```python
from build123d import *

# Parameters (mm, degrees)
SKETCH1_W                                     = 1219.2
SKETCH1_H                                     = 1778
SKETCH1_R                                     = 254
SKETCH1_W_2                                   = 361.95
SKETCH1_H_2                                   = 361.95
BOSS_EXTRUDE1_DEPTH                           = 6.35
SKETCH3_R                                     = 209.55
CUT_EXTRUDE2_DEPTH                            = 7.35
SKETCH2_W                                     = 203.2
SKETCH2_H                                     = 165.1
CUT_EXTRUDE1_DEPTH                            = 7.35
SKETCH4_R                                     = 3.3655
CUT_EXTRUDE3_DEPTH                            = 7.35
LPATTERN1_COUNT                               = 5
LPATTERN1_PITCH                               = 425.45
SKETCH5_R                                     = 3.429
CUT_EXTRUDE4_DEPTH                            = 7.35
LPATTERN2_COUNT                               = 3
LPATTERN2_PITCH                               = 301.625
SKETCH6_R                                     = 3.96875
CUT_EXTRUDE5_DEPTH                            = 7.35
SKETCH7_R                                     = 3.3782
CUT_EXTRUDE6_DEPTH                            = 7.35
CSK_FOR_1_4_FLAT_HEAD_MACHINE_SCREW1_AT_COUNT = 2
CSK_FOR_1_4_FLAT_HEAD_MACHINE_SCREW1_AT_PITCH = 63.5
LPATTERN3_COUNT                               = 2
LPATTERN3_PITCH                               = 901.7
SKETCH12_R                                    = 4.7625
CUT_EXTRUDE7_DEPTH                            = 7.35
SKETCH14_R                                    = 4.7625
CUT_EXTRUDE8_DEPTH                            = 7.35
SKETCH15_R                                    = 4.7625
CUT_EXTRUDE9_DEPTH                            = 7.35
SKETCH16_R                                    = 4.7625
CUT_EXTRUDE10_DEPTH                           = 7.35
FILLET1_R                                     = 12.7
FILLET2_R                                     = 6.35
SKETCH17_R                                    = 3.937
CUT_EXTRUDE11_DEPTH                           = 7.35
CSK_FOR_1_4_FLAT_HEAD_MACHINE_SCREW2_AT_COUNT = 2
CSK_FOR_1_4_FLAT_HEAD_MACHINE_SCREW2_AT_PITCH = 95.25
CSK_FOR_1_4_FLAT_HEAD_MACHINE_SCREW2_2_COUNT  = 2
CSK_FOR_1_4_FLAT_HEAD_MACHINE_SCREW2_2_PITCH  = 381
CSK_FOR_1_4_FLAT_HEAD_MACHINE_SCREW2_3_COUNT  = 2
CSK_FOR_1_4_FLAT_HEAD_MACHINE_SCREW2_3_PITCH  = 392.72581084
F_5_16_0_3125_DIAMETER_HOLE1_D                = 7.9375


with BuildPart() as part:
    # Sketch1 → Boss-Extrude1 (new body)
    with BuildSketch(Plane.XY):
        with Locations((609.6, 889)):
            Rectangle(SKETCH1_W, SKETCH1_H)
        with Locations((330.2, 1473.2)):
            Circle(SKETCH1_R, mode=Mode.SUBTRACT)
        with Locations((609.6, 917.575)):
            Rectangle(SKETCH1_W_2, SKETCH1_H_2, mode=Mode.SUBTRACT)
    extrude(amount=BOSS_EXTRUDE1_DEPTH)

    # Sketch3 → Cut-Extrude2 (cut, through all)
    with BuildSketch(Plane.XY.offset(6.35)):
        with Locations((609.6, 279.4)):
            Circle(SKETCH3_R)
    extrude(amount=-CUT_EXTRUDE2_DEPTH, mode=Mode.SUBTRACT)

    # Sketch2 → Cut-Extrude1 (cut, through all)
    with BuildSketch(Plane.XY.offset(6.35)):
        with Locations((609.6, 44.45)):
            Rectangle(SKETCH2_W, SKETCH2_H)
        with Locations((609.6, 514.35)):
            Rectangle(SKETCH2_W, SKETCH2_H)
    extrude(amount=-CUT_EXTRUDE1_DEPTH, mode=Mode.SUBTRACT)

    # Sketch4 → Cut-Extrude3 (cut, through all)
    with BuildSketch(Plane.XY.offset(6.35)):
        with Locations((50.8, 12.7)):
            Circle(SKETCH4_R)
    cut_extrude3 = extrude(amount=-CUT_EXTRUDE3_DEPTH, mode=Mode.SUBTRACT)

    # LPattern1: Cut-Extrude3 ×5
    with Locations(*[(0, i * LPATTERN1_PITCH, 0) for i in range(1, LPATTERN1_COUNT)]):
        add(cut_extrude3, mode=Mode.SUBTRACT)

    # Sketch5 → Cut-Extrude4 (cut, through all)
    with BuildSketch(Plane.XY.offset(6.35)):
        with Locations((609.6, 1714.5)):
            Circle(SKETCH5_R)
    cut_extrude4 = extrude(amount=-CUT_EXTRUDE4_DEPTH, mode=Mode.SUBTRACT)

    # LPattern2: Cut-Extrude4 ×3
    with Locations(*[(0, -i * LPATTERN2_PITCH, 0) for i in range(1, LPATTERN2_COUNT)]):
        add(cut_extrude4, mode=Mode.SUBTRACT)

    # Sketch6 → Cut-Extrude5 (cut, through all)
    with BuildSketch(Plane.XY.offset(6.35)):
        with Locations((127, 12.7)):
            Circle(SKETCH6_R)
        with Locations((381, 12.7)):
            Circle(SKETCH6_R)
    extrude(amount=-CUT_EXTRUDE5_DEPTH, mode=Mode.SUBTRACT)

    # Sketch7 → Cut-Extrude6 (cut, through all)
    with BuildSketch(Plane.XY.offset(6.35)):
        with Locations((777.605208253, 88.9)):
            Circle(SKETCH7_R)
        with Locations((898.525, 342.9)):
            Circle(SKETCH7_R)
        with Locations((898.525, 215.9)):
            Circle(SKETCH7_R)
    extrude(amount=-CUT_EXTRUDE6_DEPTH, mode=Mode.SUBTRACT)

    # Sketch11 → CSK for 1/4 Flat Head Machine Screw1 (revolve, cut)
    with BuildSketch(Plane(origin=(127, 85.725, 6.35), x_dir=(0, -1, 0), z_dir=(1, 0, 0))):
        Polygon((0, 0), (0, 6.35), (3.57124, 6.35), (3.57124, 3.298865467), (6.4389, 0), align=None)
    csk_for_1_4_flat_head_machine_screw1 = revolve(axis=Axis((127, 85.725, 12.7), (0, 0, -1)), mode=Mode.SUBTRACT)

    # CSK for 1/4 Flat Head Machine Screw1 at: CSK for 1/4 Flat Head Machine Screw1 ×2
    with Locations(*[(i * CSK_FOR_1_4_FLAT_HEAD_MACHINE_SCREW1_AT_PITCH, 0, 0) for i in range(1, CSK_FOR_1_4_FLAT_HEAD_MACHINE_SCREW1_AT_COUNT)]):
        add(csk_for_1_4_flat_head_machine_screw1, mode=Mode.SUBTRACT)

    # LPattern3: CSK for 1/4 Flat Head Machine Screw1 ×2
    with Locations(*[(i * LPATTERN3_PITCH, 0, 0) for i in range(1, LPATTERN3_COUNT)]):
        add(csk_for_1_4_flat_head_machine_screw1, mode=Mode.SUBTRACT)

    # LPattern3 copy 1 sketch → LPattern3 copy 1 (revolve, cut)
    with BuildSketch(Plane(origin=(1092.2, 85.725, 6.35), x_dir=(0, -1, 0), z_dir=(1, 0, 0))):
        Polygon((0, 0), (0, 6.35), (3.57124, 6.35), (3.57124, 3.298865467), (6.4389, 0), align=None)
    revolve(axis=Axis((1092.2, 85.725, 12.7), (0, 0, -1)), mode=Mode.SUBTRACT)

    # Sketch12 → Cut-Extrude7 (cut, through all)
    with BuildSketch(Plane.XY.offset(6.35)):
        with Locations((203.2, 1727.2)):
            Circle(SKETCH12_R)
        with Locations((1016, 1727.2)):
            Circle(SKETCH12_R)
    extrude(amount=-CUT_EXTRUDE7_DEPTH, mode=Mode.SUBTRACT)

    # Sketch14 → Cut-Extrude8 (cut, through all)
    with BuildSketch(Plane.XY.offset(6.35)):
        with Locations((31.75, 1651)):
            Circle(SKETCH14_R)
        with Locations((31.75, 914.4)):
            Circle(SKETCH14_R)
        with Locations((31.75, 304.8)):
            Circle(SKETCH14_R)
    cut_extrude8 = extrude(amount=-CUT_EXTRUDE8_DEPTH, mode=Mode.SUBTRACT)

    # Mirror1: Cut-Extrude8 across plane
    add(cut_extrude8.mirror(Plane.ZY.offset(-609.6)), mode=Mode.SUBTRACT)

    # Sketch15 → Cut-Extrude9 (cut, through all)
    with BuildSketch(Plane.XY.offset(6.35)):
        with Locations((403.225, 736.6)):
            Circle(SKETCH15_R)
        with Locations((403.225, 682.625)):
            Circle(SKETCH15_R)
    cut_extrude9 = extrude(amount=-CUT_EXTRUDE9_DEPTH, mode=Mode.SUBTRACT)

    # Mirror2: Cut-Extrude9 across plane
    add(cut_extrude9.mirror(Plane.ZY.offset(-609.6)), mode=Mode.SUBTRACT)

    # Sketch16 → Cut-Extrude10 (cut, through all)
    with BuildSketch(Plane.XY.offset(6.35)):
        with Locations((419.1, 1054.1)):
            Circle(SKETCH16_R)
        with Locations((419.1, 787.4)):
            Circle(SKETCH16_R)
        with Locations((800.1, 1054.1)):
            Circle(SKETCH16_R)
        with Locations((800.1, 787.4)):
            Circle(SKETCH16_R)
    extrude(amount=-CUT_EXTRUDE10_DEPTH, mode=Mode.SUBTRACT)

    # Fillet1
    fillet1_edges = [part.edges().sort_by_distance(p)[0] for p in [
        (508, 0, 3.175),
        (711.2, 0, 3.175),
    ]]
    fillet(fillet1_edges, radius=FILLET1_R)

    # Fillet2
    fillet2_edges = [part.edges().sort_by_distance(p)[0] for p in [
        (428.625, 1098.55, 3.175),
        (428.625, 736.6, 3.175),
        (790.575, 736.6, 3.175),
        (790.575, 1098.55, 3.175),
        (711.2, 596.9, 3.175),
        (508, 596.9, 3.175),
        (0, 0, 3.175),
        (1219.2, 0, 3.175),
    ]]
    fillet(fillet2_edges, radius=FILLET2_R)

    # Sketch17 → Cut-Extrude11 (cut, through all)
    with BuildSketch(Plane.XY.offset(6.35)):
        with Locations((416.56762, 76.2)):
            Circle(SKETCH17_R)
        with Locations((416.56762, 19.05)):
            Circle(SKETCH17_R)
        with Locations((797.56762, 19.05)):
            Circle(SKETCH17_R)
        with Locations((797.56762, 76.2)):
            Circle(SKETCH17_R)
    extrude(amount=-CUT_EXTRUDE11_DEPTH, mode=Mode.SUBTRACT)

    # Sketch21 → CSK for 1/4 Flat Head Machine Screw2 (revolve, cut)
    with BuildSketch(Plane(origin=(418.15512, 576.972045059, 6.35), x_dir=(0, -1, 0), z_dir=(1, 0, 0))):
        Polygon((0, 0), (0, 6.35), (3.57124, 6.35), (3.57124, 3.298865467), (6.4389, 0), align=None)
    csk_for_1_4_flat_head_machine_screw2 = revolve(axis=Axis((418.15512, 576.972045059, 12.7), (0, 0, -1)), mode=Mode.SUBTRACT)

    # CSK for 1/4 Flat Head Machine Screw2 at: CSK for 1/4 Flat Head Machine Screw2 ×2
    with Locations(*[(0, -i * CSK_FOR_1_4_FLAT_HEAD_MACHINE_SCREW2_AT_PITCH, 0) for i in range(1, CSK_FOR_1_4_FLAT_HEAD_MACHINE_SCREW2_AT_COUNT)]):
        add(csk_for_1_4_flat_head_machine_screw2, mode=Mode.SUBTRACT)

    # CSK for 1_4 Flat Head Machine Screw2 2: CSK for 1/4 Flat Head Machine Screw2 ×2
    with Locations(*[(i * CSK_FOR_1_4_FLAT_HEAD_MACHINE_SCREW2_2_PITCH, 0, 0) for i in range(1, CSK_FOR_1_4_FLAT_HEAD_MACHINE_SCREW2_2_COUNT)]):
        add(csk_for_1_4_flat_head_machine_screw2, mode=Mode.SUBTRACT)

    # CSK for 1_4 Flat Head Machine Screw2 3: CSK for 1/4 Flat Head Machine Screw2 ×2
    with Locations(*[Vector(0.9701425, -0.242535625, 0) * (i * CSK_FOR_1_4_FLAT_HEAD_MACHINE_SCREW2_3_PITCH) for i in range(1, CSK_FOR_1_4_FLAT_HEAD_MACHINE_SCREW2_3_COUNT)]):
        add(csk_for_1_4_flat_head_machine_screw2, mode=Mode.SUBTRACT)

    # 5/16 (0.3125) Diameter Hole1 (through all)
    with Locations(Plane.XY.offset(6.35)):
        with Locations((334.9625, 68.2625), (334.9625, 14.2875), (884.2375, 14.2875), (884.2375, 68.2625)):
            Hole(F_5_16_0_3125_DIAMETER_HOLE1_D / 2)


solid = part.part
```
For this review, take the finished solid that the model builds, in its own axes (mm). A direction names the side the tool comes from. Round coordinates to 2 decimals unless told otherwise and drop trailing zeros. Write each question's results on one line, items separated by ' | '.
Item 1: Draft analysis for pull direction Y (two halves, no side actions). For faces 1 (the face through (400.073, 282.523, 3.219)), 2 (the face through (601, 704, 6.35)), state which applies: pulls with the +Y half, pulls with the -Y half, needs draft (parallel to the pull), parting line crosses it, or undercut.
Calculated:
face 1: undercut | face 2: needs draft
Item 2: For pin 1 (1.9 mm diameter, centred on x = 584.5, z = 3.5, fed in from -Y); pin 2 (11.5 mm diameter, centred on x = 418.16, y = 576.97, fed in from +Z), all flat-tipped, find the tip position at first contact; note any pin that passes through.
Calculated:
pin 1: stops at y = 596.9 | pin 2: stops at z = 5.56
Item 3: For faces 3 (the face through (819.127, 276.277, 3.219)), 4 (the face through (601, 704, 0)), list the 3-axis set-ups (+Z, -Z, +X, -X, +Y, -Y) from which the entire face can be reached by the end or side of a thin tool; tool diameter is ignored.
Calculated:
face 3: +Z, -Z | face 4: -Z, +X, -X, +Y, -Y
Item 4: Take a section at A-A on z = 5.25. Count the separate pieces of the cut face and the enclosed holes in it, then the cut area to 3 significant figures.
Calculated:
separate pieces: 1 | enclosed holes: 47 | area: 1,650,000 mm^2
Item 5: To check wall thickness, follow line 1 along X through (y, z) = (787.4, 2.25) (1 decimal); line 2 along X through (y, z) = (836, 4.75) (3 decimals); line 3 along Y through (x, z) = (1028.7, 1.7). State the ranges of each line that lie inside material, in increasing order. Write a range as from..to.
Calculated:
line 1: x = 0..414.3, 423.9..428.6, 790.6..795.3, 804.9..1219.2 | line 2: x = 0..428.625, 790.575..1219.2 | line 3: y = 0..82.15, 89.3..1778
